Design review of the part built by this model. Coordinates are the model's own, in mm. A direction names the side the tool comes from. Coordinates: 2 decimals unless noted, no trailing zeros. Order: outer loops, then holes, each group sorted by start corner. A loop starts at its lowest first (then second) coordinate and runs counter-clockwise, first axis right, second up. Notation, with made-up numbers: (10, 66) -> (64, 66) arc R26 cw to (64, 100) -> close; hole circle Ø4 at (-20, 89.5). An arc over 180 degrees is marked (long way). Write item = value, one per line.
```python
from build123d import *

# Parameters (mm, degrees)
SKETCH1_W           = 76.2
SKETCH1_H           = 25.4
BOSS_EXTRUDE1_DEPTH = 12.7
SKETCH2_W           = 19.05
SKETCH2_H           = 6.35
CUT_EXTRUDE1_DEPTH  = 82.319677815
CUT_EXTRUDE2_DEPTH  = 3.175
FILLET1_R           = 1.27


with BuildPart() as part:
    # Sketch1 → Boss-Extrude1 (new body)
    with BuildSketch(Plane(origin=(0, 0, 0), x_dir=(1, 0, 0), z_dir=(0, 1, 0))):
        with Locations((38.1, 12.7)):
            Rectangle(SKETCH1_W, SKETCH1_H)
    extrude(amount=BOSS_EXTRUDE1_DEPTH)

    # Sketch2 → Cut-Extrude1 (cut, through all)
    with BuildSketch(Plane(origin=(76.2, 0, 0), x_dir=(0, 0, -1), z_dir=(1, 0, 0))):
        with Locations((12.7, 6.35)):
            Rectangle(SKETCH2_W, SKETCH2_H)
    extrude(amount=-CUT_EXTRUDE1_DEPTH, mode=Mode.SUBTRACT)

    # Sketch3 → Cut-Extrude2 (cut)
    with BuildSketch(Plane(origin=(0, 12.7, 0), x_dir=(1, 0, 0), z_dir=(0, 1, 0))):
        with BuildLine():
            Line((12.573, 6.35), (63.627, 6.35))
            ThreePointArc((63.627, 6.35), (68.027325499, 8.172674501), (69.85, 12.573))
            Line((69.85, 12.573), (69.85, 12.827))
            ThreePointArc((69.85, 12.827), (68.027325499, 17.227325499), (63.627, 19.05))
            Line((63.627, 19.05), (12.573, 19.05))
            ThreePointArc((12.573, 19.05), (8.172674501, 17.227325499), (6.35, 12.827))
            Line((6.35, 12.827), (6.35, 12.573))
            ThreePointArc((6.35, 12.573), (8.172674501, 8.172674501), (12.573, 6.35))
        make_face()
    extrude(amount=-CUT_EXTRUDE2_DEPTH, mode=Mode.SUBTRACT)

    # Fillet1
    fillet1_edges = [part.edges().sort_by_distance(p)[0] for p in [
        (0, 6.35, -25.4),
        (76.2, 6.35, -25.4),
        (76.2, 6.35, 0),
        (0, 6.35, 0),
    ]]
    fillet(fillet1_edges, radius=FILLET1_R)


solid = part.part
```
(1) We need section D-D (y = 11.25). Write out the cut boundary in (x, z), and give its area (3 significant figures).
Report:
outline = (0, -24.13) arc R1.27 ccw to (1.27, -25.4) -> (74.93, -25.4) arc R1.27 ccw to (76.2, -24.13) -> (76.2, -1.27) arc R1.27 ccw to (74.93, 0) -> (1.27, 0) arc R1.27 ccw to (0, -1.27) -> close; hole (6.35, -12.83) arc R6.22 ccw to (12.57, -19.05) -> (63.63, -19.05) arc R6.22 ccw to (69.85, -12.83) -> (69.85, -12.57) arc R6.22 ccw to (63.63, -6.35) -> (12.57, -6.35) arc R6.22 ccw to (6.35, -12.57) -> close
area = 1,160 mm²
(2) We need section B-B (y = 6.75). Write out the cut boundary in (x, z) (3 decimals), and give its area (3 significant figures).
Report:
outline = (0, -24.13) arc R1.27 ccw to (1.27, -25.4) -> (74.93, -25.4) arc R1.27 ccw to (76.2, -24.13) -> (76.2, -22.225) -> (0, -22.225) -> close; (0, -3.175) -> (76.2, -3.175) -> (76.2, -1.27) arc R1.27 ccw to (74.93, 0) -> (1.27, 0) arc R1.27 ccw to (0, -1.27) -> close
area = 482 mm²
(3) The part is to be moulded in two halves that separate along X. For faces 1 (the cylindrical face through (8.221, 11.135, -17.275)), 2 (the flat face through (38, 11, -6.35)), 3 (the flat face through (76.2, 2, -13)), 4 (the flat face through (39, 6, -3.175)), say which applies: released by +X, released by -X, zero draft, split by the parting line, or undercut.
Report:
face_1 = undercut
face_2 = undercut
face_3 = released by +X
face_4 = zero draft
(4) For faces 5 (the flat face through (38, 6, 0)), 6 (the flat face through (39, 6, -22.225)), 7 (the cylindrical face through (8.125, 11.135, -8.221)), list the 3-axis set-ups (+Z, -Z, +X, -X, +Y, -Y) from which the entire face can be reached by the end or side of a thin tool; tool diameter is ignored.
Report:
face_5 = +Z, +X, -X, +Y, -Y
face_6 = +X, -X
face_7 = +Y
(5) Insertion check: pin 1 (5.5 mm diameter, centred on x = 42.5, z = -11.5, fed in from +Y) (3 decimals). The pin has a flat end and moves straight along its axis. Give the tip position at first contact, or say it passes through.
Report:
pin_1 = 3.175
(6) For L1, parallel to Z at x = 38.5, y = 7 (3 decimals); L2, parallel to Z at x = 36, y = 10; L3, parallel to Y at x = 25.5, z = -4.75 (3 decimals), list the stretches that pass through material, from the lowest coordinate up.
Report:
L1 = -25.4 to -22.225, -3.175 to 0
L2 = -25.4 to -19.05, -6.35 to 0
L3 = 0 to 3.175, 9.525 to 12.7
(7) We need section C-C (z = -16.25). Write out the cut boundary in (x, y) (3 decimals), and give its area (3 significant figures).
Report:
outline = (0, 0) -> (76.2, 0) -> (76.2, 3.175) -> (0, 3.175) -> close; (0, 9.525) -> (7.376, 9.525) -> (7.376, 12.7) -> (0, 12.7) -> close; (68.824, 9.525) -> (76.2, 9.525) -> (76.2, 12.7) -> (68.824, 12.7) -> close
area = 289 mm²
(8) We need section A-A (x = 26.5). Write out the cut boundary in (y, z) (3 decimals), and give its area (3 significant figures).
Report:
outline = (0, -25.4) -> (12.7, -25.4) -> (12.7, -19.05) -> (9.525, -19.05) -> (9.525, -22.225) -> (3.175, -22.225) -> (3.175, -3.175) -> (9.525, -3.175) -> (9.525, -6.35) -> (12.7, -6.35) -> (12.7, 0) -> (0, 0) -> close
area = 161 mm²
